Read the model definition and answer for the solid it produces. Units are mm, in the model's axes. Coordinates: 2 decimals unless noted, no trailing zeros. Order: outer loops, then holes, each group sorted by start corner. A loop starts at its lowest first (then second) coordinate and runs counter-clockwise, first axis right, second up. Notation, with made-up numbers: M 33.5,40.25 L 37.5,40.25 A20 ccw 37.5,52.25 Z; hole C 38,11 d7. An arc over 180 degrees is marked long. One line per question, with ' | ' between items. Start each with the question number.
1) Given P1, Ø1, axis at y = 0, z = -2, coming from the +X side; P2, Ø0.5, axis at x = -9, z = -0.5, coming from the +Y side; P3, Ø1.5, axis at x = 6, z = 5, coming from the +Y side; P4, Ø1.1, axis at y = 0, z = -1.81, coming from the -X side, each flat-ended and moving along its own axis, determine where each tip first touches the part or whether it passes through.
2) Find section D-D, the plane z = 34. Write down the section's boundary in (x, y).
3) Consider probe 1 along Z at (x, y) = (11, -4.25); probe 2 along Z at (x, y) = (9.35, 0); probe 3 along Y at (x, z) = (6.5, 19). Determine where each line is inside the solid, lowest interval first.
4) Find section C-C, the plane y = 9.5. Write down the section's boundary in (x, z), plus the area to 3 significant figures.
5) Find section B-B, the plane z = 24.5. Write down the section's boundary in (x, y).
6) Find section A-A, the plane x = 0. Write down the section's boundary in (y, z), plus the area to 3 significant figures.
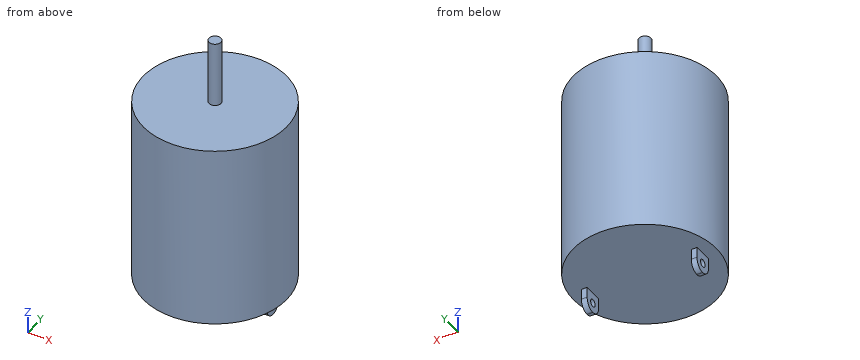
from build123d import *

# Parameters (mm, degrees)
F0_R     = 12
F1_DEPTH = 31
F2_R     = 1
F3_DEPTH = 11
F4_W     = 0.961760059
F4_H     = 3.1858317088
F5_DEPTH = 3.5
F6_R     = 0.6249075308
F7_DEPTH = 21.7267718444


with BuildPart() as f1:
    # F0 (on Top) → F1 (new body)
    with BuildSketch(Plane.XY):
        Circle(F0_R)
    extrude(amount=F1_DEPTH)

    # F2 (on face) → F3 (join)
    with BuildSketch(Plane.XY.offset(31)):
        Circle(F2_R)
    extrude(amount=F3_DEPTH)

    # F4 (on face) → F5 (join)
    with BuildSketch(Plane(origin=(0, 0, 0), x_dir=(1, 0, 0), z_dir=(0, 0, -1))):
        with Locations((-9.2448918149, -0.0064170454)):
            Rectangle(F4_W, F4_H)
        with Locations((9.2448918149, -0.0064170454)):
            Rectangle(F4_W, F4_H)
    extrude(amount=F5_DEPTH)

    # F6 (on face) → F7 (cut, through all)
    with BuildSketch(Plane.YZ.offset(9.7257718444)):
        with BuildLine():
            add(Edge.make_bspline(
                [(0.0887662493, -3.5), (0.8568494058, -3.4783165811), (1.5993328998, -2.8509894263), (1.5993328998, -1.75)],
                knots=[0.5172392132, 0.5172392132, 0.5172392132, 0.5172392132, 1, 1, 1, 1], degree=3))
            Line((0.0887662493, -3.5), (1.5993328998, -3.5))
            Line((1.5993328998, -3.5), (1.5993328998, -1.75))
        make_face()
        with BuildLine():
            add(Edge.make_bspline(
                [(-1.586498809, -1.75), (-1.586498809, -2.800242044), (-0.7900408818, -3.4774841708), (0.0064170454, -3.5)],
                knots=[0, 0, 0, 0, 0.5, 0.5, 0.5, 0.5], degree=3))
            Line((-1.586498809, -1.75), (-1.586498809, -3.5))
            Line((-1.586498809, -3.5), (0.0064170454, -3.5))
        make_face()
        with Locations((0, -1.8095459091)):
            Circle(F6_R)
    extrude(amount=-F7_DEPTH, mode=Mode.SUBTRACT)


solid = f1.part
Report:
1) P1: stops at x = 9.73 | P2: stops at y = 1.6 | P3: stops at y = 10.79 | P4: passes through
2) outline: C 0,0 d2
3) probe 1: z = 0 to 31 | probe 2: z = -3.5 to -2.43, -1.18 to 31 | probe 3: y = -10.09 to 10.09
4) outline: M -7.33,0 L 7.33,0 L 7.33,31 L -7.33,31 Z | area: 455 mm^2
5) outline: C 0,0 d24
6) outline: M -12,0 L 12,0 L 12,31 L 1,31 L 1,42 L -1,42 L -1,31 L -12,31 Z | area: 766 mm^2
